Source: CAD feature listing. Evaluate the final solid. Frame: model axes, mm. A direction names the side the tool comes from. Coordinates: 2 decimals unless noted, no trailing zeros. Order: outer loops, then holes, each group sorted by start corner. A loop starts at its lowest first (then second) coordinate and runs counter-clockwise, first axis right, second up.
Item 1: Section C-C on y = 0. Return the cut outline in (x, z), then the cut area to 3 significant figures.
Item 2: Reachability of faces 4 (the flat face through (2, 0, -3)), 5 (the flat face through (0, 24, 0)), 6 (the cylindrical face through (0.5, 0.18, 4.18)) from +Z, -Z, +X, -X, +Y, -Y: full face, straight path, thin tool, end or side. Return the list, or none.
Item 3: Contact query for flat-ended pins moving along their axis: P1, Ø3, axis at y = 2.5, z = -3.5, coming from the +X side; P2, Ø2.5, axis at x = 3.5, y = 1, coming from the +Z side. Output: stop coordinate, or through.
Item 4: Section A-A on x = 5.5. Return the cut outline in (y, z), then the cut area to 3 significant figures.
Item 5: Section D-D on x = 2. Return the cut outline in (y, z), then the cut area to 3 significant figures.
Item 6: Mould query, pull axis Y, two halves, no side actions, for faces 1 (the flat face through (2, 0, 2.3)), 2 (the flat face through (8.5, -15, 0)), 3 (the flat face through (0, -24, 0)). Classes: released by +Y, released by -Y, zero draft, split by the parting line, or undercut.
Item 7: Ray query, line 1 (Z direction, x = 7.5, y = 7); line 2 (Y direction, x = 5.25, z = 3.75); line 3 (Y direction, x = 7.75, z = -2). Return the intervals inside material, ascending.
from build123d import *

# Parameters (mm, degrees)
PAD_DEPTH       = 6
POCKET_DEPTH    = 3.7
POCKET001_DEPTH = 3


with BuildPart() as part:
    # Sketch → Pad (new body, symmetric)
    with BuildSketch(Plane.XY):
        with BuildLine():
            Line((8.5, 24), (-8.5, 24))
            Line((-8.5, 24), (-8.5, -24))
            Line((-8.5, -24), (8.500003, -24))
            Line((8.500003, -24), (8.500003, -6))
            ThreePointArc((8.5, 6), (2.500003, -1e-06), (8.500003, -6))
            Line((8.5, 24), (8.5, 6))
        make_face()
    extrude(amount=PAD_DEPTH, both=True)

    # Sketch001 → Pocket (cut)
    with BuildSketch(Plane.XY.offset(6)):
        with BuildLine():
            ThreePointArc((8.5, 8), (0.499974, 1.3e-05), (8.499974, -8))
            Line((24.499948, -8), (8.499974, -8))
            Line((24.499948, 7.999948), (24.499948, -8))
            Line((8.5, 8), (24.499948, 7.999948))
        make_face()
    extrude(amount=-POCKET_DEPTH, mode=Mode.SUBTRACT)

    # Sketch002 → Pocket001 (cut)
    with BuildSketch(Plane(origin=(0, 0, -6), x_dir=(1, 0, 0), z_dir=(0, 0, -1))):
        with BuildLine():
            ThreePointArc((8.5, 8), (0.499986, 7e-06), (8.499985, -8))
            Line((24.499971, -8), (8.499985, -8))
            Line((24.499971, 7.999971), (24.499971, -8))
            Line((8.5, 8), (24.499971, 7.999971))
        make_face()
    extrude(amount=-POCKET001_DEPTH, mode=Mode.SUBTRACT)


solid = part.part
Answer list:
1. outline: (-8.5, -6) - (0.5, -6) - (0.5, -3) - (2.5, -3) - (2.5, 2.3) - (0.5, 2.3) - (0.5, 6) - (-8.5, 6) - close
1. area: 119 mm2
2. face 4: -Z, +X
2. face 5: +Z, -Z, +X, -X, +Y
2. face 6: +Z, +X
3. P1: stops at x = 3.95
3. P2: stops at z = 2.3
4. outline: (-24, -6) - (-7.42, -6) - (-7.42, -3) - (-5.2, -3) - (-5.2, 2.3) - (-7.42, 2.3) - (-7.42, 6) - (-24, 6) - close; (5.2, -3) - (7.42, -3) - (7.42, -6) - (24, -6) - (24, 6) - (7.42, 6) - (7.42, 2.3) - (5.2, 2.3) - close
4. area: 422 mm2
5. outline: (-24, -6) - (-4.66, -6) - (-4.66, -3) - (4.66, -3) - (4.66, -6) - (24, -6) - (24, 6) - (4.66, 6) - (4.66, 2.3) - (-4.66, 2.3) - (-4.66, 6) - (-24, 6) - close
5. area: 514 mm2
6. face 1: undercut
6. face 2: zero draft
6. face 3: released by -Y
7. line 1: z = -3 to 2.3
7. line 2: y = -24 to -7.31, 7.31 to 24
7. line 3: y = -24 to -5.95, 5.95 to 24
